Geometry: final body of the model. Coordinates: model frame, mm. A direction names the side the tool comes from. Give positions to 0.01 mm unless a question says otherwise; leave off trailing zeros. Order: outer loops, then holes, each group sorted by start corner. A loop starts at its lowest first (then second) coordinate and runs counter-clockwise, first axis right, second up. Notation, with made-up numbers: (76, -4.5) - (87, -4.5) arc R11 ccw to (87, 16.5) - close; hole circle Ø2 at (-16.75, -38.5). An arc over 180 degrees is marked (long way). One line per item, written item: value.
```python
from build123d import *

# Parameters (mm, degrees)
SKETCH1_W                  = 17
SKETCH1_H                  = 17
BOSS_EXTRUDE1_DEPTH        = 20
SHELL1_T                   = -1.8
F_6_5_6_5_DIAMETER_HOLE1_D = 6.5
SKETCH5_W                  = 5
SKETCH5_H                  = 15.022252834
CUT_EXTRUDE1_DEPTH         = 4


with BuildPart() as part:
    # Sketch1 → Boss-Extrude1 (new body)
    with BuildSketch(Plane(origin=(0, 0, 0), x_dir=(1, 0, 0), z_dir=(0, 1, 0))):
        with Locations((8.5, 8.5)):
            Rectangle(SKETCH1_W, SKETCH1_H)
    extrude(amount=BOSS_EXTRUDE1_DEPTH)

    # Shell1
    shell1_openings = [part.faces().sort_by_distance(p)[0] for p in [
        (8.5, 20, -8.5),
    ]]
    offset(amount=SHELL1_T, openings=shell1_openings, kind=Kind.INTERSECTION)

    # Ø6.5 (6.5) Diameter Hole1 (through all)
    with Locations(Plane(origin=(0, 0, 0), x_dir=(-1, 0, 0), z_dir=(0, -1, 0))):
        with Locations((-8.5, 8.5)):
            Hole(F_6_5_6_5_DIAMETER_HOLE1_D / 2)

    # Sketch5 → Cut-Extrude1 (cut)
    with BuildSketch(Plane.ZY):
        with Locations((-8.5, 12.488873583)):
            Rectangle(SKETCH5_W, SKETCH5_H)
    extrude(amount=-CUT_EXTRUDE1_DEPTH, mode=Mode.SUBTRACT)


solid = part.part
```
1) First-contact query: pin 1 (5 mm diameter, centred on x = 7.5, z = -9, fed in from +Y); pin 2 (1 mm diameter, centred on y = 6, z = -8, fed in from -X); pin 3 (2 mm diameter, centred on x = 1, z = -8.5, fed in from +Y). Flat tips, straight axial feed; report the tip coordinate or a pass-through.
Answers below:
pin 1: y = 1.8
pin 2: x = 15.2
pin 3: y = 4.98
2) Section C-C, the plane y = 4.25. Return loops of the section in (x, z).
Answers below:
outline: (0, -17) - (17, -17) - (17, 0) - (0, 0) - close; hole (1.8, -15.2) - (15.2, -15.2) - (15.2, -1.8) - (1.8, -1.8) - close
3) Section D-D, the plane y = 18.5. Return loops of the section in (x, z), then the cut area to 3 significant figures.
Answers below:
outline: (0, -17) - (17, -17) - (17, 0) - (0, 0) - (0, -6) - (1.8, -6) - (1.8, -1.8) - (15.2, -1.8) - (15.2, -15.2) - (1.8, -15.2) - (1.8, -11) - (0, -11) - close
area: 100 mm^2
4) Section B-B, the plane x = 8.5. Return loops of the section in (y, z).
Answers below:
outline: (0, -17) - (20, -17) - (20, -15.2) - (1.8, -15.2) - (1.8, -11.75) - (0, -11.75) - close; (0, -5.25) - (1.8, -5.25) - (1.8, -1.8) - (20, -1.8) - (20, 0) - (0, 0) - close
5) Material intervals for line 1 along Z through (x, y) = (15, 18.75); line 2 along X through (y, z) = (1.4, -8.5); line 3 along Z through (x, y) = (8.5, 1.2), sorted ascending.
Answers below:
line 1: -17 to -15.2, -1.8 to 0
line 2: 0 to 5.25, 11.75 to 17
line 3: -17 to -11.75, -5.25 to 0
6) Set-up query: faces 1 (the face through (1, 12, -6)), 2 (the face through (8, 10, 0)), 3 (the face through (8, 11, -15.2)). Return all of +Z, -Z, +X, -X, +Y, -Y with unobstructed straight access to the full face (end or side cutting, diameter ignored); none if empty.
Answers below:
face 1: -X, +Y
face 2: +Z, +X, -X, +Y, -Y
face 3: +Y
7) Section A-A, the plane z = -8.5. Return loops of the section in (x, y).
Answers below:
outline: (0, 0) - (5.25, 0) - (5.25, 1.8) - (1.8, 1.8) - (1.8, 4.98) - (0, 4.98) - close; (11.75, 0) - (17, 0) - (17, 20) - (15.2, 20) - (15.2, 1.8) - (11.75, 1.8) - close
8) Mould query, pull axis X, two halves, no side actions, for faces 4 (the face through (1, 4.978, -9)), 5 (the face through (1.8, 11, -5)), 6 (the face through (17, 10, -8)), 7 (the face through (0, 10, -12)). Classes: released by +X, released by -X, zero draft, split by the parting line, or undercut.
Answers below:
face 4: zero draft
face 5: undercut
face 6: released by +X
face 7: released by -X
